Autodesk Inventor part; units mm, degrees
ref_plane "YZ Plane" through (0, 0, 0) normal (1, 0, 0) x (0, 1, 0)
ref_plane "XZ Plane" through (0, 0, 0) normal (0, 1, 0) x (-1, 0, 0)
ref_plane "XY Plane" through (0, 0, 0) normal (0, 0, 1) x (1, 0, 0)
sketch "Sketch1" plane through (0, 0, 0) normal (0, 0, 1) x (1, 0, 0)
  line L0 (0, 0) -> (5.5, 0)
  line L1 (5.5, 0) -> (5.5, 37)
  line L2 (5.5, 37) -> (0, 37)
  line L3 (0, 37) -> (0, 0)
  line L4 (0, 0) -> (5.5, 0)
  line L5 (5.5, 0) -> (5.5, 37)
  line L6 (5.5, 37) -> (0, 37)
  line L7 (0, 37) -> (0, 0)
  line L8 (0, 0) -> (5.5, 0)
  line L9 (5.5, 0) -> (5.5, 37)
  line L10 (5.5, 37) -> (0, 37)
  line L11 (0, 37) -> (0, 0)
  line L12 (0, 0) -> (5.5, 0)
  line L13 (5.5, 0) -> (5.5, 37)
  line L14 (5.5, 37) -> (0, 37)
  line L15 (0, 37) -> (0, 0)
  point P0 (2.75, 34)
  point P1 (2.75, 3)
  point P2 (2.75, 34)
  point P3 (2.75, 3)
  point P4 (2.75, 34)
  point P5 (2.75, 3)
  point P6 (2.75, 34)
  point P7 (2.75, 3)
  dimension "d0" = 5.5
  dimension "d1" = 37
  dimension "d2" = 3
  dimension "d3" = 2.75
  dimension "d4" = 3
  dimension "d5" = 5.5
  dimension "d6" = 37
  dimension "d7" = 3
  dimension "d8" = 2.75
  dimension "d9" = 3
  dimension "d10" = 5.5
  dimension "d11" = 37
  dimension "d12" = 3
  dimension "d13" = 2.75
  dimension "d14" = 3
  dimension "d15" = 5.5
  dimension "d16" = 37
  dimension "d17" = 3
  dimension "d18" = 2.75
  dimension "d19" = 3
extrude "Extrusion1" add sketch "Sketch1" along normal blind 17
sketch "Sketch2" plane through (0, 0, 0) normal (0, 0, 1) x (1, 0, 0)
  line L0 (0, 0) -> (5.5, 0)
  line L1 (5.5, 0) -> (5.5, 37)
  line L2 (5.5, 37) -> (0, 37)
  line L3 (0, 37) -> (0, 0)
  line L4 (0, 0) -> (5.5, 0)
  line L5 (5.5, 0) -> (5.5, 37)
  line L6 (5.5, 37) -> (0, 37)
  line L7 (0, 37) -> (0, 0)
  line L8 (0, 0) -> (5.5, 0)
  line L9 (5.5, 0) -> (5.5, 37)
  line L10 (5.5, 37) -> (0, 37)
  line L11 (0, 37) -> (0, 0)
  line L12 (0, 0) -> (5.5, 0)
  line L13 (5.5, 0) -> (5.5, 37)
  line L14 (5.5, 37) -> (0, 37)
  line L15 (0, 37) -> (0, 0)
  point P0 (2.75, 34)
  point P1 (2.75, 3)
  point P2 (2.75, 34)
  point P3 (2.75, 3)
  point P4 (2.75, 34)
  point P5 (2.75, 3)
  point P6 (2.75, 34)
  point P7 (2.75, 3)
  dimension "d20" = 5.5
  dimension "d21" = 37
  dimension "d22" = 3
  dimension "d23" = 2.75
  dimension "d24" = 3
  dimension "d25" = 5.5
  dimension "d26" = 37
  dimension "d27" = 3
  dimension "d28" = 2.75
  dimension "d29" = 3
  dimension "d30" = 5.5
  dimension "d31" = 37
  dimension "d32" = 3
  dimension "d33" = 2.75
  dimension "d34" = 3
  dimension "d35" = 5.5
  dimension "d36" = 37
  dimension "d37" = 3
  dimension "d38" = 2.75
  dimension "d39" = 3
hole "Hole1" at (2.75, 34, 0) at (2.75, 3, 0) direction (0, 0, 1) diameter 3.5 end through all
sketch "Sketch3" plane through (5.5, 0, 0) normal (1, 0, 0) x (0, 0, -1)
  line L0 (0, 0) -> (-17, 0)
  line L1 (-17, 0) -> (1, 0)
  line L2 (1, 0) -> (1, 37)
  line L3 (1, 37) -> (-17, 37)
  line L4 (-17, 37) -> (-17, 0)
  arc A0 (1, 31.125) -> (1, 5.875) centre (1, 18.5) ccw
  dimension "d49" = 18
  dimension "d50" = 25.25
extrude "Extrusion2" cut sketch "Sketch3" against normal blind 5.5 contours A0 L2
properties part number "SujetadorColaVTOLv2"
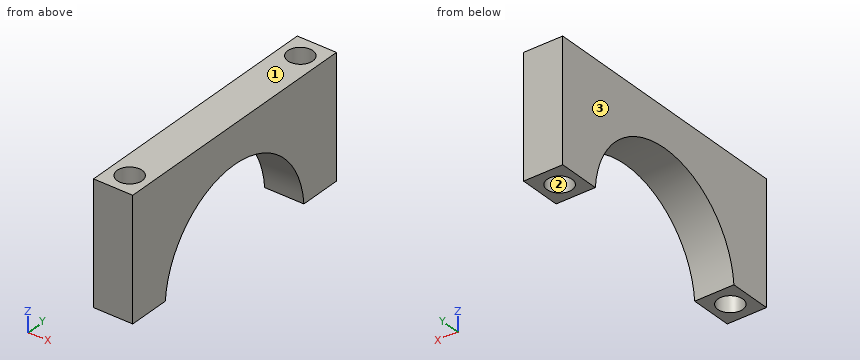
For this review, take the finished solid that the model builds, in its own axes (mm). Face numbers are marked on the shaded views. Round coordinates to 2 decimals unless told otherwise and drop trailing zeros. Order: outer loops, then holes, each group sorted by start corner. A loop starts at its lowest first (then second) coordinate and runs counter-clockwise, first axis right, second up. Notation, with made-up numbers: M 79,-37 L 110,-37 A16 cw 110,-23 Z; hole C -9,83.25 d5. An arc over 180 degrees is marked long. Use a Markdown table: item, result. Add a question column.
Item 1: Insertion check: pin 1 (1.5 mm diameter, centred on x = 2.5, z = 12, fed in from -Y); pin 2 (3 mm diameter, centred on x = 2.75, y = 3, fed in from -Z). Each pin has a flat end and moves straight along its axis. Give the tip position at first contact, or say it passes through.
Item 2: Add section C-C, the plane z = 11. Give the boundary of the cut face in (x, y), then the cut area to 3 significant figures.
Item 3: Add section A-A, the plane x = 2.75. Give the boundary of the cut face in (y, z) (3 decimals), then the cut area to 3 significant figures.
Item 4: Add section B-B, the plane y = 34. Give the boundary of the cut face in (x, z).
Item 5: Mouldability with a two-part tool opening along X and no side actions: class the marked faces 1, 2 and 3 as released by +X, released by -X, zero draft, split by the parting line, or undercut.
Item 6: Add section D-D, the plane z = 4.5. Give the boundary of the cut face in (x, y).
Item 7: To check wall thickness, follow line 1 along Y through (x, z) = (2.75, 13.25); line 2 along X through (y, z) = (34, 10.5); line 3 along Y through (x, z) = (2.75, 7.25). State the ranges of each line that lie inside material, in increasing order.
Geometry results:
| question | item | result |
|---|---|---|
| 1 | pin 1 | stops at y = 0 |
| 1 | pin 2 | passes through |
| 2 | outline | M 0,0 L 5.5,0 L 5.5,14.58 L 0,14.58 Z; M 0,22.42 L 5.5,22.42 L 5.5,37 L 0,37 Z; hole C 2.75,3 d3.5; hole C 2.75,34 d3.5 |
| 2 | area | 141 mm² |
| 3 | outline | M 0,0 L 1.25,0 L 1.25,17 L 0,17 Z; M 4.75,0 L 5.915,0 A12.625 cw 31.085,0 L 32.25,0 L 32.25,17 L 4.75,17 Z; M 35.75,0 L 37,0 L 37,17 L 35.75,17 Z |
| 3 | area | 285 mm² |
| 4 | outline | M 0,0 L 1,0 L 1,17 L 0,17 Z; M 4.5,0 L 5.5,0 L 5.5,17 L 4.5,17 Z |
| 5 | face 1 | zero draft |
| 5 | face 2 | undercut |
| 5 | face 3 | released by -X |
| 6 | outline | M 0,0 L 5.5,0 L 5.5,7.14 L 0,7.14 Z; M 0,29.86 L 5.5,29.86 L 5.5,37 L 0,37 Z; hole C 2.75,3 d3.5; hole C 2.75,34 d3.5 |
| 7 | line 1 | y = 0 to 1.25, 4.75 to 32.25, 35.75 to 37 |
| 7 | line 2 | x = 0 to 1, 4.5 to 5.5 |
| 7 | line 3 | y = 0 to 1.25, 4.75 to 8.94, 28.06 to 32.25, 35.75 to 37 |
